```python
from build123d import *

# Parameters (mm, degrees)
ESQUISSE1_R             = 1.6
BOSS_EXTRU_1_DEPTH      = 3
ESQUISSE2_R             = 1.5
ENL_V_MAT_EXTRU_1_DEPTH = 10


with BuildPart() as part:
    # Esquisse1 → Boss.-Extru.1 (new body)
    with BuildSketch(Plane.XY):
        with BuildLine():
            Line((2.16040571, 38.470971764), (37.868700226, 3.47214746))
            ThreePointArc((37.868700226, 3.47214746), (39.068592938, 0.655617594), (37.925457843, -2.184422046))
            Line((37.925457843, -2.184422046), (2.926633539, -37.892716563))
            ThreePointArc((2.926633539, -37.892716563), (0.110103674, -39.092609274), (-2.729935967, -37.94947418))
            Line((-2.729935967, -37.94947418), (-38.438230483, -2.950649875))
            ThreePointArc((-38.438230483, -2.950649875), (-39.638123195, -0.13412001), (-38.4949881, 2.705919631))
            Line((-38.4949881, 2.705919631), (-3.496163796, 38.414214147))
            ThreePointArc((-3.496163796, 38.414214147), (-0.67963393, 39.614106858), (2.16040571, 38.470971764))
        make_face()
        with Locations((10.790147704, 3.13130948)):
            Circle(ESQUISSE1_R, mode=Mode.SUBTRACT)
        with Locations((-3.720649665, -9.530710886)):
            Circle(ESQUISSE1_R, mode=Mode.SUBTRACT)
        with Locations((32.240509529, 0.58710509)):
            Circle(ESQUISSE1_R, mode=Mode.SUBTRACT)
        Polygon((16.69738986, -7.699410262), (8.297672026, -16.269400946), (-8.128143451, -0.169941765), (0.271574382, 8.400048919), align=None, mode=Mode.SUBTRACT)
    extrude(amount=BOSS_EXTRU_1_DEPTH)

    # Esquisse2 → Enlèv. mat.-Extru.1 (cut)
    with BuildSketch(Plane(origin=(0, 0, 0), x_dir=(-1, 0, 0), z_dir=(0, 0, -1))):
        with Locations((0.820879588, 36.0721308)):
            Circle(ESQUISSE2_R)
        with Locations((35.95969919, 0.221003105)):
            Circle(ESQUISSE2_R)
        with Locations((-0.141386567, -35.162808267)):
            Circle(ESQUISSE2_R)
    extrude(amount=-ENL_V_MAT_EXTRU_1_DEPTH, mode=Mode.SUBTRACT)


solid = part.part
```
Work out the finished part from the listing and answer in its coordinate system (mm). A direction names the side the tool comes from. Round coordinates to 2 decimals unless told otherwise and drop trailing zeros. Order: outer loops, then holes, each group sorted by start corner. A loop starts at its lowest first (then second) coordinate and runs counter-clockwise, first axis right, second up.
Q1. A tool of negligible diameter and unlimited length cuts with its end or side. For faces 4 (the flat face through (9, 1, 3)), 5 (the flat face through (8.37, 0.46, 1.48)), from which of +Z, -Z, +X, -X, +Y, -Y can it reach the whole face along a straight path? Write none if from no direction.
Solution:
face 4: +Z, +X, -X, +Y, -Y
face 5: +Z, -Z
Q2. Given pin 1 Ø8 at (x, y) = (-30.5, 16) entering from +Z, flat-ended and moving along its own axis, determine where the tip first touches the part or whether it passes through.
Solution:
pin 1: stops at z = 3
Q3. A cutting plane is placed at C-C, the plane x = -7. Determine the outline of the cut face in (y, z), then the cut area to 3 significant figures.
Solution:
outline: (-33.76, 0) - (-1.28, 0) - (-1.28, 3) - (-33.76, 3) - close; (0.98, 0) - (34.84, 0) - (34.84, 3) - (0.98, 3) - close
area: 199 mm2
Q4. The mould has two halves that part along X. Classify faces 1 (the cylindrical face through (0.154, -39.092, 1.479)), 2 (the cylindrical face through (31.06, 1.67, 1.48)), 3 (the flat face through (19.76, 21.22, 1.48)): pulls with the +X half, pulls with the -X half, needs draft (parallel to the pull), parting line crosses it, or undercut.
Solution:
face 1: parting line crosses it
face 2: undercut
face 3: pulls with the +X half
Q5. A cutting plane is placed at B-B, the plane z = 1.45. Determine the outline of the cut face in (x, y).
Solution:
outline: (-38.49, 2.71) arc R4 ccw to (-38.44, -2.95) - (-2.73, -37.95) arc R4 ccw to (2.93, -37.89) - (37.93, -2.18) arc R4 ccw to (37.87, 3.47) - (2.16, 38.47) arc R4 ccw to (-3.5, 38.41) - close; hole circle Ø3 at (-35.96, 0.22); hole (-8.13, -0.17) - (8.3, -16.27) - (16.7, -7.7) - (0.27, 8.4) - close; hole circle Ø3.2 at (-3.72, -9.53); hole circle Ø3 at (-0.82, 36.07); hole circle Ø3 at (0.14, -35.16); hole circle Ø3.2 at (10.79, 3.13); hole circle Ø3.2 at (32.24, 0.59)
Q6. Find the intervals of material crossed by line 1 along Y through (x, z) = (-2, 2.65); line 2 along Y through (x, z) = (11.5, 2.5); line 3 along X through (y, z) = (-9.5, 1.7), in increasing order.
Solution:
line 1: y = -38.52 to -6.18, 6.08 to 35.14, 37 to 39.38
line 2: y = -29.15 to -13, -2.61 to 1.7, 4.57 to 29.32
line 3: x = -31.76 to -5.32, -2.12 to 1.39, 14.93 to 30.76
Q7. A cutting plane is placed at D-D, the plane y = 30. Determine the outline of the cut face in (x, z), then the cut area to 3 significant figures.
Solution:
outline: (-11.74, 0) - (10.8, 0) - (10.8, 3) - (-11.74, 3) - close
area: 67.6 mm2
Q8. A cutting plane is placed at A-A, the plane x = 4.5. Determine the outline of the cut face in (y, z).
Solution:
outline: (-36.29, 0) - (-12.55, 0) - (-12.55, 3) - (-36.29, 3) - close; (4.26, 0) - (36.18, 0) - (36.18, 3) - (4.26, 3) - close
